```python
from build123d import *

# Parameters (mm, degrees)
F1_DEPTH = 3
F3_DEPTH = 5
F4_R     = 2.49999


# Not quite as in the source:
# - a fillet or chamfer is up to 0.001 mm smaller than in the source, because OpenCascade refuses the exact size


with BuildPart() as f1:
    # F0 (on Top) → F1 (new body)
    with BuildSketch(Plane.XY):
        with BuildLine():
            ThreePointArc((0, 2.5), (1.767766953, 1.767766953), (2.5, 0))
            ThreePointArc((2.5, 0), (1.767766953, -1.767766953), (0, -2.5))
            Line((0, -2.5), (4.8989794856, -2.5))
            ThreePointArc((4.8989794856, -2.5), (5.3476343915, -1.2856151892), (5.5, 0))
            ThreePointArc((5.5, 0), (5.3476343915, 1.2856151892), (4.8989794856, 2.5))
            Line((4.8989794856, 2.5), (0, 2.5))
        make_face()
        with BuildLine():
            ThreePointArc((0, -2.5), (-2.5, 0), (0, 2.5))
            Line((0, 2.5), (4.8989794856, 2.5))
            ThreePointArc((4.8989794856, 2.5), (-5.5, 0), (4.8989794856, -2.5))
            Line((4.8989794856, -2.5), (0, -2.5))
        make_face()
        with BuildLine():
            Line((8.5, 2.5), (4.8989794856, 2.5))
            ThreePointArc((4.8989794856, 2.5), (5.3476343915, 1.2856151892), (5.5, 0))
            ThreePointArc((5.5, 0), (5.3476343915, -1.2856151892), (4.8989794856, -2.5))
            Line((4.8989794856, -2.5), (8.5, -2.5))
            Line((8.5, -2.5), (8.5, 2.5))
        make_face()
    extrude(amount=F1_DEPTH)

    # F2 (on face) → F3 (join, through all)
    with BuildSketch(Plane.XZ.offset(2.5)):
        with BuildLine():
            Line((2.5, 5), (4.6270166538, 5))
            ThreePointArc((4.6270166538, 5), (6.0505102572, 7.1622776602), (8.5, 8))
            Line((8.5, 8), (2.5, 8))
            Line((2.5, 8), (2.5, 5))
        make_face()
        with BuildLine():
            Line((8.5, 0), (8.5, 3))
            Line((8.5, 3), (4.8989794856, 3))
            Line((4.8989794856, 3), (4.8989794856, 2.258549095))
            ThreePointArc((4.8989794856, 2.258549095), (6.3746533953, 0.6113569368), (8.5, 0))
        make_face()
        with BuildLine():
            ThreePointArc((8.5, 5), (9.2071067812, 4.7071067812), (9.5, 4))
            ThreePointArc((9.5, 4), (9.2071067812, 3.2928932188), (8.5, 3))
            Line((8.5, 3), (8.5, 0))
            ThreePointArc((8.5, 0), (11.3284271247, 1.1715728753), (12.5, 4))
            ThreePointArc((12.5, 4), (11.3284271247, 6.8284271247), (8.5, 8))
            ThreePointArc((8.5, 8), (6.0505102572, 7.1622776602), (4.6270166538, 5))
            Line((4.6270166538, 5), (8.5, 5))
        make_face()
    extrude(amount=-F3_DEPTH)

    # F4 (radius 2.5 in the source; OpenCascade refuses exactly that, so slightly less here)
    f4_edges = [f1.edges().sort_by_distance(p)[0] for p in [
        (2.5, -2.5, 6.5),
        (2.5, 2.5, 6.5),
    ]]
    fillet(f4_edges, radius=F4_R)


solid = f1.part
```
Model file for the job. Use its own axes, mm. A direction names the side the tool comes from. Give positions to 0.01 mm unless a question says otherwise; leave off trailing zeros. Write each loop counter-clockwise with the first axis right and the second up, starting at its lowest first coordinate (ties: lowest second). Pieces come first, ordered by that corner, then holes. Notation, with made-up numbers: M 56,20.25 L 73,20.25 A9 ccw 73,28.25 Z; hole C 24.25,-7 d7. An arc over 180 degrees is marked long. Use a Markdown table: item, result.
1) Cut at B-B (z = 2.25). List the corners of the cut face in (x, y), and give its area (3 significant figures).
Responses:
| item | result |
|---|---|
| outline | M 4.9,-2.5 L 12.1,-2.5 L 12.1,2.5 L 4.9,2.5 A5.5 ccw long Z; hole C 0,0 d5 |
| area | 109 mm2 |
2) Drill centre lines: line 1 (Z direction, x = 8.25, y = 2); line 2 (Y direction, x = 9.5, z = 1.5); line 3 (Y direction, x = 0, z = 0.75). Where is each one in solid material? Low to high. Write a range as from..to.
Responses:
| item | result |
|---|---|
| line 1 | z = 0..3, 5..8 |
| line 2 | y = -2.5..2.5 |
| line 3 | y = -5.5..-2.5, 2.5..5.5 |
3) Cut at A-A (y = -1.75). List the corners of the cut face in (x, z).
Responses:
| item | result |
|---|---|
| outline | M -5.21,0 L -1.79,0 L -1.79,3 L -5.21,3 Z; M 1.79,0 L 8.5,0 A4 ccw 8.5,8 L 3.21,8 L 3.21,5 L 8.5,5 A1 cw 8.5,3 L 1.79,3 Z |
4) Tool access for faces 5 (the flat face through (9.5, -2.5, 3.2)), 6 (the cylindrical face through (3.252, 1.787, 6.479)), 7 (the cylindrical face through (3.252, -1.787, 6.479)), 8 (the flat face through (9.5, 2.5, 3.2)), 9 (the cylindrical face through (-5.496, 0.206, 1.479)): list every direction of +Z, -Z, +X, -X, +Y, -Y with a clear straight run to the whole face (end or side of a thin tool).
Responses:
| item | result |
|---|---|
| face 5 | +Z, -Z, +X, -Y |
| face 6 | +Z, -X, +Y |
| face 7 | +Z, -X, -Y |
| face 8 | +Z, -Z, +X, +Y |
| face 9 | +Z, -Z |
5) Pull direction Z, two halves, no side cores. Call faces 1 (the flat face through (5, 0, 5)), 2 (the flat face through (3, 0, 0)), 3 (the flat face through (6, 0, 8)), 4 (the flat face through (3, 0, 3)): +Z half, -Z half, draft (parallel to the pull), parting line (faces both ways), or undercut.
Responses:
| item | result |
|---|---|
| face 1 | undercut |
| face 2 | -Z half |
| face 3 | +Z half |
| face 4 | undercut |
6) Cut at C-C (x = -2). List the corners of the cut face in (y, z), and give its area (3 significant figures).
Responses:
| item | result |
|---|---|
| outline | M -5.12,0 L -1.5,0 L -1.5,3 L -5.12,3 Z; M 1.5,0 L 5.12,0 L 5.12,3 L 1.5,3 Z |
| area | 21.7 mm2 |
7) Pin check, flat tips, straight feed: pin 1 (1.5 mm diameter, centred on x = -2.5, y = 0, fed in from +Z); pin 2 (1.5 mm diameter, centred on y = 3.5, z = 3, fed in from -X); pin 3 (1.5 mm diameter, centred on x = 4.5, y = 0.5, fed in from -Z); pin 4 (3 mm diameter, centred on x = 8.5, z = 5.5, fed in from +Y). Stop position of each tip, or through.
Responses:
| item | result |
|---|---|
| pin 1 | stops at z = 3 |
| pin 2 | stops at x = -4.76 |
| pin 3 | stops at z = 0 |
| pin 4 | stops at y = 2.5 |
